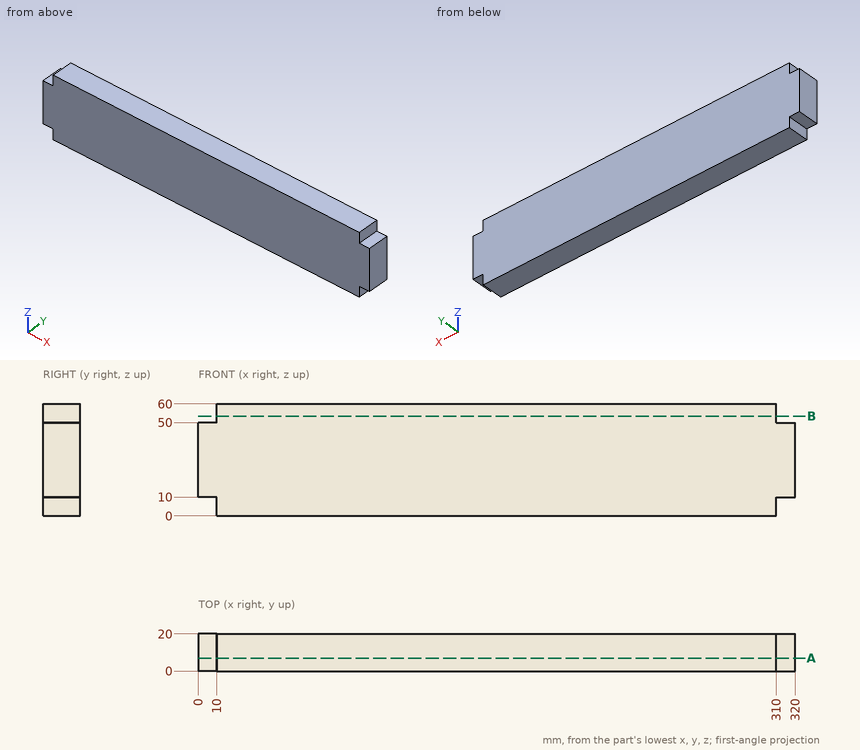
Here's the drawing with two shaded views (mm, measured from the low corner). I have some questions. Round coordinates to 2 decimals unless told otherwise and drop trailing zeros. Order: outer loops, then holes, each group sorted by start corner. A loop starts at its lowest first (then second) coordinate and runs counter-clockwise, first axis right, second up. Notation, with made-up numbers: (28, 78) -> (35, 78) arc R26 cw to (35, 97) -> close; hole circle Ø6 at (51, 28.5). An arc over 180 degrees is marked (long way). Use a Markdown table: item, result. Add a question column.
(1) I need wall thicknesses on line 1 along X through (y, z) = (8, 55). Which ranges of the line are inside material? Lowest first, please.
(2) Suppose I cut it at B-B, the plane z = 53.5. Please give me the cut outline in (x, y).
(3) Suppose I cut it at A-A, the plane y = 7. Please give me the cut outline in (x, z).
(4) For pin 1 Ø8 at (x, y) = (4.5, 9) entering from -Z; pin 2 Ø3 at (y, z) = (11.5, 56.5) entering from +X; pin 3 Ø11 at (y, z) = (9, 56.5) entering from -X, each with a flat end and sliding along its axis, tell me the tip position at first contact or that it passes through.
Verdict:
| question | item | result |
|---|---|---|
| 1 | line 1 | 10 to 310 |
| 2 | outline | (10, 0) -> (310, 0) -> (310, 20) -> (10, 20) -> close |
| 3 | outline | (0, 10) -> (10, 10) -> (10, 0) -> (310, 0) -> (310, 10) -> (320, 10) -> (320, 50) -> (310, 50) -> (310, 60) -> (10, 60) -> (10, 50) -> (0, 50) -> close |
| 4 | pin 1 | z = 10 |
| 4 | pin 2 | x = 310 |
| 4 | pin 3 | x = 10 |
